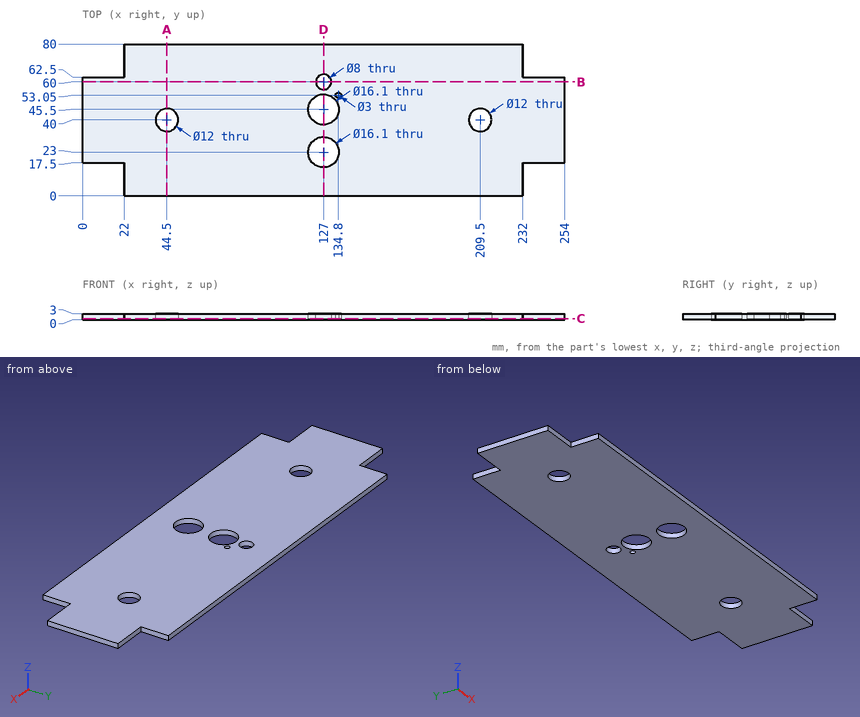
Can you work these out from the drawing? Everything is in mm from the part's minimum corner. Round coordinates to 2 decimals unless told otherwise and drop trailing zeros. Order: outer loops, then holes, each group sorted by start corner. A loop starts at its lowest first (then second) coordinate and runs counter-clockwise, first axis right, second up. Notation, with made-up numbers: (52, -13.5) -> (89, -13.5) arc R24 cw to (89, 23.5) -> close; hole circle Ø7 at (-37, 11). An arc over 180 degrees is marked (long way). Return JSON: item names as keys, results as strings. Group by question number.
1. I need wall thicknesses on line 1 (Y direction, x = 127, z = 0.8); line 2 (Y direction, x = 209.5, z = 1.4); line 3 (Y direction, x = 120, z = 2.85). Which ranges of each line are inside material? Lowest first, please. Write a range as [from, to].
2. If we section it at D-D, the plane x = 127: Write out the boundary of the cut face in (y, z), then the cut area to 3 significant figures.
3. If we section it at B-B, the plane y = 60: Write out the boundary of the cut face in (x, z), then the cut area to 3 significant figures.
4. If we section it at C-C, the plane z = 0.5: Write out the boundary of the cut face in (x, y).
5. Will these pins go through, and if not, where does the flat tip stop? pin 1 (9.5 mm diameter, centred on x = 127, y = 45.5, fed in from +Z); pin 2 (1.5 mm diameter, centred on y = 69.5, z = 2, fed in from +X); pin 3 (1.5 mm diameter, centred on y = 12, z = 2, fed in from -X); pin 4 (1.5 mm diameter, centred on x = 9, z = 1.5, fed in from -Y).
6. If we section it at A-A, the plane x = 44.5: Write out the boundary of the cut face in (y, z).
Output values:
{
 "1": {"line 1": "[0, 14.95], [31.05, 37.45], [53.55, 56], [64, 80]", "line 2": "[0, 34], [46, 80]", "line 3": "[0, 19.02], [26.98, 41.52], [49.48, 80]"},
 "2": {"outline": "(0, 0) -> (14.95, 0) -> (14.95, 3) -> (0, 3) -> close; (31.05, 0) -> (37.45, 0) -> (37.45, 3) -> (31.05, 3) -> close; (53.55, 0) -> (56, 0) -> (56, 3) -> (53.55, 3) -> close; (64, 0) -> (80, 0) -> (80, 3) -> (64, 3) -> close", "area": "119 mm²"},
 "3": {"outline": "(0, 0) -> (123, 0) -> (123, 3) -> (0, 3) -> close; (131, 0) -> (254, 0) -> (254, 3) -> (131, 3) -> close", "area": "738 mm²"},
 "4": {"outline": "(0, 17.5) -> (22, 17.5) -> (22, 0) -> (232, 0) -> (232, 17.5) -> (254, 17.5) -> (254, 62.5) -> (232, 62.5) -> (232, 80) -> (22, 80) -> (22, 62.5) -> (0, 62.5) -> close; hole circle Ø12 at (44.5, 40); hole circle Ø16.1 at (127, 23); hole circle Ø16.1 at (127, 45.5); hole circle Ø8 at (127, 60); hole circle Ø3 at (134.8, 53.05); hole circle Ø12 at (209.5, 40)"},
 "5": {"pin 1": "through", "pin 2": "x = 232", "pin 3": "x = 22", "pin 4": "y = 17.5"},
 "6": {"outline": "(0, 0) -> (34, 0) -> (34, 3) -> (0, 3) -> close; (46, 0) -> (80, 0) -> (80, 3) -> (46, 3) -> close"}
}
